Check sheet for the modelled part. Datum: model origin and axes. Units: mm. A direction names the side the tool comes from. Round coordinates to 2 decimals unless told otherwise and drop trailing zeros. Loops run counter-clockwise (first coordinate to the right, second up) from the corner with the lowest first, then second, coordinate; pieces in that order, holes last. Notation, with made-up numbers: M -14,8.5 L 14,8.5 A32 ccw 14,43.5 Z; hole C 44,44 d5. An arc over 180 degrees is marked long. Write item = value, one per line. Start each with the question number.
(1) Scan lines: L1, parallel to Y at x = 8, z = 6.5; L2, parallel to Z at x = -48, y = 40. Record each from-to range of solid material in increasing order. Write a range as from..to.
(2) Cross-section at A-A on y = -40. Record the boundary of the cut face in (x, z), plus the area to 3 significant figures.
(3) Go/stop test with flat-tipped pins: P1, Ø4.5, axis at y = -40, z = 5, coming from the -X side; P2, Ø1, axis at x = -7.5, y = 19, coming from the +Z side. Record where each tip stops, or that it passes through.
(4) Mould release check, pull along Z, two halves, no side actions. Record for faces 4 (the face through (50, -1, 5)), 5 (the face through (-1, 1, 5)), 6 (the face through (-45, -40, 4)): pulls with the +Z half, pulls with the -Z half, needs draft (parallel to the pull), parting line crosses it, or undercut.
(5) Cross-section at D-D on z = 12. Record the boundary of the cut face in (x, y).
(6) Cross-section at B-B on x = -21. Record the boundary of the cut face in (y, z).
(7) Set-up check for faces 1 (the face through (-45, 40, 4)), 2 (the face through (-1, 50, 5)), 3 (the face through (46.3, -48.4, 12.2)): record each of +Z, -Z, +X, -X, +Y, -Y from which the full face is reachable in a straight line by a thin tool's end or side.
from build123d import *

# Parameters (mm, degrees)
F0_W     = 100
F0_H     = 100
F1_DEPTH = 10
F2_T     = -5
F3_R     = 1.499724
F3_R_2   = 1.5
F3_R_3   = 1.400261
F4_DEPTH = 5
F5_SIZE  = 0.5
F6_R     = 2.5
F7_DEPTH = 5


with BuildPart() as f1:
    # F0 (on Top) → F1 (new body)
    with BuildSketch(Plane.XY):
        Rectangle(F0_W, F0_H)
    extrude(amount=F1_DEPTH)

    # F2
    f2_openings = [f1.faces().sort_by_distance(p)[0] for p in [
        (0, 0, 10),
    ]]
    offset(amount=F2_T, openings=f2_openings)

    # F3 (on face) → F4 (join)
    with BuildSketch(Plane.XY.offset(10)):
        with Locations((-47.5, -47.5)):
            Circle(F3_R)
        with Locations((47.5, -47.5)):
            Circle(F3_R_2)
        with Locations((47.5, 47.5)):
            Circle(F3_R_3)
        with Locations((-47.5, 47.5)):
            Circle(F3_R_2)
    extrude(amount=F4_DEPTH)

    # F5
    f5_edges = [f1.edges().sort_by_distance(p)[0] for p in [
        (46.099739, 47.5, 15),
        (-49, 47.5, 15),
        (-48.999724, -47.5, 15),
        (46, -47.5, 15),
    ]]
    chamfer(f5_edges, length=F5_SIZE)

    # F6 (on face) → F7 (cut)
    with BuildSketch(Plane(origin=(-50, 0, 0), x_dir=(0, -1, 0), z_dir=(-1, 0, 0))):
        with Locations((40, 5)):
            Circle(F6_R)
        with Locations((-40, 5)):
            Circle(F6_R)
    extrude(amount=-F7_DEPTH, mode=Mode.SUBTRACT)


solid = f1.part
Result:
q1.L1 = -50..-45, 45..50
q1.L2 = 0..2.5, 7.5..10
q2.outline = M -50,0 L 50,0 L 50,10 L 45,10 L 45,5 L -45,5 L -45,2.5 L -50,2.5 Z; M -50,7.5 L -45,7.5 L -45,10 L -50,10 Z
q2.area = 525 mm^2
q3.P1 = -45
q3.P2 = 5
q4.face_4 = needs draft
q4.face_5 = pulls with the +Z half
q4.face_6 = undercut
q5.outline = C -47.5,-47.5 d3; C -47.5,47.5 d3; C 47.5,-47.5 d3; C 47.5,47.5 d2.8
q6.outline = M -50,0 L 50,0 L 50,10 L 45,10 L 45,5 L -45,5 L -45,10 L -50,10 Z
q7.face_1 = -X
q7.face_2 = +Z, -Z, +X, -X, +Y
q7.face_3 = +Z
